The listing builds one solid part. Answer for the finished solid, in the listing's coordinates (mm). Face numbers are marked on the shaded views. Coordinates: 2 decimals unless noted, no trailing zeros. Order: outer loops, then holes, each group sorted by start corner. A loop starts at its lowest first (then second) coordinate and runs counter-clockwise, first axis right, second up.
from build123d import *

# Parameters (mm, degrees)
SKETCH_1_W          = 20
SKETCH_1_H          = 20
SKETCH_1_R          = 1.65
EXTRUDE_1_DEPTH     = 5
SKETCH_2_W          = 20
SKETCH_2_H          = 1
CUT_EXTRUDE_1_DEPTH = 5


with BuildPart() as part:
    # 草图1 → 凸台-拉伸1 (new body)
    with BuildSketch(Plane.XY):
        Rectangle(SKETCH_1_W, SKETCH_1_H)
        with Locations((-5, 0)):
            Circle(SKETCH_1_R, mode=Mode.SUBTRACT)
        with Locations(Location((5, 0, 0), (0, 0, 180))):
            Circle(SKETCH_1_R, mode=Mode.SUBTRACT)
    extrude(amount=EXTRUDE_1_DEPTH)

    # 草图2 → 切除-拉伸1 (cut)
    with BuildSketch(Plane.XY.offset(5)):
        with Locations((0, 9.5)):
            Rectangle(SKETCH_2_W, SKETCH_2_H)
    extrude(amount=-CUT_EXTRUDE_1_DEPTH, mode=Mode.SUBTRACT)


solid = part.part
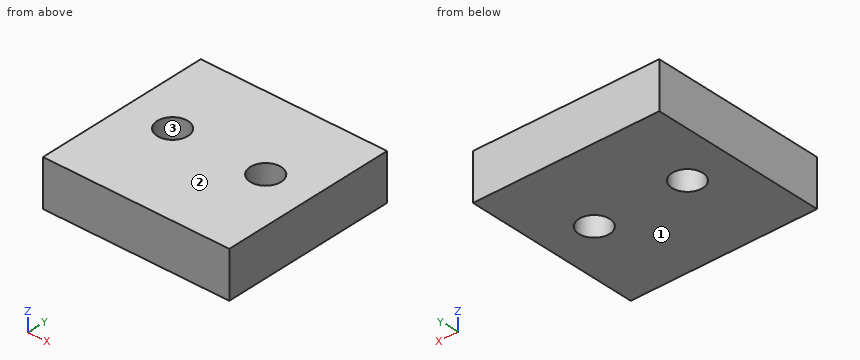
(1) The mould has two halves that part along Z. Classify the marked faces 1, 2 and 3: pulls with the +Z half, pulls with the -Z half, needs draft (parallel to the pull), parting line crosses it, or undercut.
(2) Find section C-C on z = 2.6. Determine the outline of the cut face in (x, y).
(3) Find section A-A on x = 5. Determine the outline of the cut face in (y, z), then the cut area to 3 significant figures.
(4) Find the intervals of material crossed by probe 1 along Y at (x, z) = (5, 1.7); probe 2 along Y at (x, z) = (-3.5, 0.95), in increasing order.
(5) Find section B-B on y = 0. Determine the outline of the cut face in (x, z).
Resolved:
1. face 1: pulls with the -Z half
1. face 2: pulls with the +Z half
1. face 3: needs draft
2. outline: (-10, -10) - (10, -10) - (10, 9) - (-10, 9) - close; hole circle Ø3.3 at (-5, 0); hole circle Ø3.3 at (5, 0)
3. outline: (-10, 0) - (-1.65, 0) - (-1.65, 5) - (-10, 5) - close; (1.65, 0) - (9, 0) - (9, 5) - (1.65, 5) - close
3. area: 78.5 mm2
4. probe 1: y = -10 to -1.65, 1.65 to 9
4. probe 2: y = -10 to -0.69, 0.69 to 9
5. outline: (-10, 0) - (-6.65, 0) - (-6.65, 5) - (-10, 5) - close; (-3.35, 0) - (3.35, 0) - (3.35, 5) - (-3.35, 5) - close; (6.65, 0) - (10, 0) - (10, 5) - (6.65, 5) - close
